```python
from build123d import *

# Parameters (mm, degrees)
F0_W      = 508
F0_H      = 127
F0_R      = 38.1
F1_DEPTH  = 190.5
F3_DEPTH  = 25.4
F4_R      = 12.7
F5_W      = 127
F5_H      = 127
F6_DEPTH  = 12.7
F7_W      = 127
F7_H      = 127
F8_DEPTH  = 12.7
F9_R      = 12.7
F10_DEPTH = 25.4


with BuildPart() as f1:
    # F0 (on Top) → F1 (new body)
    with BuildSketch(Plane.XY):
        with Locations((254, 63.5)):
            Rectangle(F0_W, F0_H)
        with Locations((63.5, 63.5)):
            Circle(F0_R, mode=Mode.SUBTRACT)
        with Locations((190.5, 63.5)):
            Circle(F0_R, mode=Mode.SUBTRACT)
        with Locations((317.5, 63.5)):
            Circle(F0_R, mode=Mode.SUBTRACT)
        with Locations((444.5, 63.5)):
            Circle(F0_R, mode=Mode.SUBTRACT)
    extrude(amount=-F1_DEPTH)

    # F2 (on face) → F3 (join)
    with BuildSketch(Plane(origin=(0, 0, -190.5), x_dir=(1, 0, 0), z_dir=(0, 0, -1))):
        Polygon((254, 0), (215.9, 0), (254, -38.1), align=None)
        Polygon((254, 0), (254, -38.1), (292.1, 0), align=None)
        Polygon((254, -127), (254, -88.9), (215.9, -127), align=None)
        Polygon((292.1, -127), (254, -88.9), (254, -127), align=None)
        Polygon((127, 0), (127, -38.1), (165.1, 0), align=None)
        Polygon((127, 0), (88.9, 0), (127, -38.1), align=None)
        Polygon((127, -88.9), (88.9, -127), (127, -127), align=None)
        Polygon((165.1, -127), (127, -88.9), (127, -127), align=None)
        Polygon((0, -38.1), (38.1, 0), (0, 0), align=None)
        Polygon((38.1, -127), (0, -88.9), (0, -127), align=None)
        Polygon((381, 0), (342.9, 0), (381, -38.1), align=None)
        Polygon((381, 0), (381, -38.1), (419.1, 0), align=None)
        Polygon((508, 0), (469.9, 0), (508, -38.1), align=None)
        Polygon((508, -88.9), (469.9, -127), (508, -127), align=None)
        Polygon((381, -88.9), (342.9, -127), (381, -127), align=None)
        Polygon((419.1, -127), (381, -88.9), (381, -127), align=None)
    extrude(amount=F3_DEPTH)

    # F4
    f4_edges = [f1.edges().sort_by_distance(p)[0] for p in [
        (400.05, 19.05, -215.9),
        (361.95, 19.05, -215.9),
        (488.95, 19.05, -215.9),
        (488.95, 107.95, -215.9),
        (400.05, 107.95, -215.9),
        (361.95, 107.95, -215.9),
        (273.05, 19.05, -215.9),
        (273.05, 107.95, -215.9),
        (234.95, 107.95, -215.9),
        (234.95, 19.05, -215.9),
        (146.05, 19.05, -215.9),
        (107.95, 19.05, -215.9),
        (107.95, 107.95, -215.9),
        (146.05, 107.95, -215.9),
        (19.05, 19.05, -215.9),
        (19.05, 107.95, -215.9),
        (292.1, 0, -203.2),
        (215.9, 0, -203.2),
        (292.1, 127, -203.2),
        (215.9, 127, -203.2),
        (342.9, 127, -203.2),
        (419.1, 127, -203.2),
        (469.9, 127, -203.2),
        (469.9, 0, -203.2),
        (419.1, 0, -203.2),
        (342.9, 0, -203.2),
        (88.9, 0, -203.2),
        (165.1, 0, -203.2),
        (88.9, 127, -203.2),
        (165.1, 127, -203.2),
        (38.1, 127, -203.2),
        (38.1, 0, -203.2),
    ]]
    fillet(f4_edges, radius=F4_R)

    # F5 (on face) → F6 (join)
    with BuildSketch(Plane.YZ.offset(508)):
        with Locations((63.5, -279.4)):
            Rectangle(F5_W, F5_H)
        with BuildLine():
            Line((106.8605122421, -215.9), (127, -215.9))
            Line((127, -215.9), (127, 0))
            Line((127, 0), (0, 0))
            Line((0, 0), (0, -215.9))
            Line((0, -215.9), (20.1394877579, -215.9))
            add(Edge.make_bspline(
                [(20.1394877579, -215.9), (38.1, -215.9), (38.1, -203.2)],
                knots=[4.7123889804, 4.7123889804, 4.7123889804, 6.2831853072, 6.2831853072, 6.2831853072], degree=2, weights=[1, 0.7071067812, 1]))
            Line((38.1, -203.2), (38.1, -190.5))
            Line((38.1, -190.5), (88.9, -190.5))
            Line((88.9, -190.5), (88.9, -203.2))
            add(Edge.make_bspline(
                [(88.9, -203.2), (88.9, -215.9), (106.8605122421, -215.9)],
                knots=[3.1415926536, 3.1415926536, 3.1415926536, 4.7123889804, 4.7123889804, 4.7123889804], degree=2, weights=[1, 0.7071067812, 1]))
        make_face()
    extrude(amount=F6_DEPTH)

    # F7 (on face) → F8 (join)
    with BuildSketch(Plane(origin=(0, 0, 0), x_dir=(0, -1, 0), z_dir=(-1, 0, 0))):
        with Locations((-63.5, -279.4)):
            Rectangle(F7_W, F7_H)
        with BuildLine():
            Line((-20.1394877579, -215.9), (0, -215.9))
            Line((0, -215.9), (0, 0))
            Line((0, 0), (-127, 0))
            Line((-127, 0), (-127, -215.9))
            Line((-127, -215.9), (-106.8605122421, -215.9))
            add(Edge.make_bspline(
                [(-106.8605122421, -215.9), (-88.9, -215.9), (-88.9, -203.2)],
                knots=[4.7123889804, 4.7123889804, 4.7123889804, 6.2831853072, 6.2831853072, 6.2831853072], degree=2, weights=[1, 0.7071067812, 1]))
            Line((-88.9, -203.2), (-88.9, -190.5))
            Line((-88.9, -190.5), (-38.1, -190.5))
            Line((-38.1, -190.5), (-38.1, -203.2))
            add(Edge.make_bspline(
                [(-38.1, -203.2), (-38.1, -215.9), (-20.1394877579, -215.9)],
                knots=[3.1415926536, 3.1415926536, 3.1415926536, 4.7123889804, 4.7123889804, 4.7123889804], degree=2, weights=[1, 0.7071067812, 1]))
        make_face()
    extrude(amount=F8_DEPTH)

    # F9 (on face) → F10 (cut)
    with BuildSketch(Plane.YZ.offset(520.7)):
        with Locations((63.5, -304.8)):
            Circle(F9_R)
    extrude(amount=-F10_DEPTH, mode=Mode.SUBTRACT)


solid = f1.part
```
Verification items for the finished model (mm, model axes). A direction names the side the tool comes from. Coordinates: 2 decimals unless noted, no trailing zeros. Write each loop counter-clockwise with the first axis right and the second up, starting at its lowest first coordinate (ties: lowest second). Pieces come first, ordered by that corner, then holes. Notation, with made-up numbers: (29, -13) - (70, -13) arc R17 cw to (70, 6) - close; hole circle Ø10 at (-5, 54). An arc over 180 degrees is marked (long way). One line per question, with ' | ' between items. Start each with the question number.
1. Gauge pin test, flat ends, axial feed: P1, Ø8, axis at x = 9.5, y = 13.5, coming from the -Z side; P2, Ø10, axis at x = 119.5, y = 105, coming from the -Z side. Record the tip position at first contact, or that the pin passes through.
2. Section check D-D (z = -236). Enter the section's corners in (x, y), plus the area to 3 significant figures.
3. Section check A-A (z = -304.8). Enter the section's corners in (x, y).
4. Draft check along Z on faces 5 (the flat face through (-6, 38.1, -197)), 6 (the flat face through (258, 0, -98)), 7 (the cylindrical face through (9.82, 104.12, -212.28)). Enter one of: released by +Z, released by -Z, zero draft, split by the parting line, or undercut.
5. Section check B-B (x = 317.5). Enter the section's corners in (y, z), plus the area to 3 significant figures.
6. Section check C-C (y = 63.5). Count the separate pieces of the cut face and the enclosed holes in it, plus the area to 3 significant figures.
7. Material ranges on line 1 along Z through (x, y) = (513.5, 63.5); line 2 along X through (y, z) = (81, -144.5); line 3 along X through (y, z) = (106, -270.5), recorded low to high.
8. Access from +Z, -Z, +X, -X, +Y, -Y to the whole of each face (thin tool, end or side, straight path). Record for faces 1 (the flat face through (-6, 88.9, -197)), 2 (the cylindrical face through (162.42, 89.25, -93.92)), 3 (the cylindrical face through (488.75, 118.97, -203.38)), 4 (the flat face through (6, 8, -215.9)).
Computed values:
1) P1: z = -215.9 | P2: z = -215.8
2) outline: (-12.7, 0) - (0, 0) - (0, 127) - (-12.7, 127) - close; (508, 0) - (520.7, 0) - (520.7, 127) - (508, 127) - close | area: 3,230 mm²
3) outline: (-12.7, 0) - (0, 0) - (0, 127) - (-12.7, 127) - close; (508, 0) - (520.7, 0) - (520.7, 50.8) - (508, 50.8) - close; (508, 76.2) - (520.7, 76.2) - (520.7, 127) - (508, 127) - close
4) face 5: undercut | face 6: zero draft | face 7: released by -Z
5) outline: (0, -190.5) - (25.4, -190.5) - (25.4, 0) - (0, 0) - close; (101.6, -190.5) - (127, -190.5) - (127, 0) - (101.6, 0) - close | area: 9,680 mm²
6) separate pieces: 8 | enclosed holes: 0 | area: 46,500 mm²
7) line 1: -342.9 to -317.5, -292.1 to -215.9, -190.5 to 0 | line 2: -12.7 to 29.66, 97.34 to 156.66, 224.34 to 283.66, 351.34 to 410.66, 478.34 to 520.7 | line 3: -12.7 to 0, 508 to 520.7
8) face 1: +X, -X | face 2: +Z, -Z | face 3: -Z | face 4: -Z, +Y, -Y
